Source: CAD feature listing. Evaluate the final solid. Frame: model axes, mm. A direction names the side the tool comes from. Coordinates: 2 decimals unless noted, no trailing zeros. Loops run counter-clockwise (first coordinate to the right, second up) from the corner with the lowest first, then second, coordinate; pieces in that order, holes last.
Item 1: Section query D-D, the plane z = 3. Return the cut outline in (x, y).
Item 2: Section query A-A, the plane y = -130. Return the cut outline in (x, z).
Item 3: Section query B-B, the plane x = 77. Return the cut outline in (y, z).
Item 4: Line query: probe 1 along Y at (x, z) = (110, -2.25); probe 2 along Y at (x, z) = (109.5, 4); probe 3 along X at (y, z) = (-91, 5.25). Output: solid intervals per line, ascending.
Item 5: Pin query (flat end, axial travel): pin 1 Ø2 at (y, z) = (-138, 3.5) entering from -X; pin 2 Ø3 at (x, z) = (68, -1) entering from -Y; pin 3 Ø2 at (x, z) = (124.5, -1.5) entering from +Y; pin 4 Ø0.9 at (y, z) = (-97, -1) entering from +X. Return the tip coordinate at first contact, or that it passes through.
Item 6: Reachability of faces 1 (the flat face through (2.631, -132, -1)), 2 (the flat face through (115, -136.459, 3)), 3 (the flat face through (0.631, -133, -1)), 4 (the flat face through (17, -143.959, -1)), 5 (the flat face through (128.131, -95, 3)) from +Z, -Z, +X, -X, +Y, -Y: full face, straight path, thin tool, end or side. Return the list, or none.
Item 7: Section query C-C, the plane y = -139.5. Return the cut outline in (x, z), then the cut area to 3 significant figures.
Item 8: Pull-direction query (Y, two-part tool) for faces 6 (the flat face through (13, -83.959, -1)), 7 (the flat face through (115, -116.459, 3)), 8 (the cylindrical face through (-4.307, -119.307, 3.451)); classes: +Y half, -Y half, draft (parallel to the pull), parting line (faces both ways), or undercut.
```python
from build123d import *

# Parameters (mm, degrees)
SKETCH1_W               = 29.381998836
SKETCH1_H               = 2
SKETCH1_W_2             = 22.166752634
SKETCH1_W_3             = 2
SKETCH1_H_2             = 20.351479426
SKETCH1_W_4             = 38.729480665
SKETCH1_W_5             = 32.851790847
SKETCH1_H_3             = 17.059842407
SKETCH1_H_4             = 0.5
SKETCH1_R               = 5
SKETCH1_R_2             = 1.75
BOSS_EXTRUDE1_DEPTH     = 7
BOSS_EXTRUDE3_DEPTH     = 3
CUT_EXTRUDE1_DEPTH      = 18
CUT_EXTRUDE1_DEPTH_BACK = 23
SKETCH2_R               = 8.5
SKETCH2_W               = 15
SKETCH2_H               = 20


with BuildPart() as part:
    # Sketch1 → Boss-Extrude1 (new body)
    # profile 1 of 26: a face of its own
    with BuildSketch(Plane.XY):
        Polygon((123.631337811, -141.958879214), (123.631337811, -121.052392275), (123.631337811, -103.992549868), (123.631337811, -85.958879214), (95.983128658, -85.958879214), (63.131337811, -85.958879214), (63.131337811, -141.958879214), (85.298090445, -141.958879214), align=None)
    # profile 2 of 26: a face of its own
    with BuildSketch(Plane.XY):
        Polygon((33.749338975, -141.958879214), (63.131337811, -141.958879214), (63.131337811, -85.958879214), (24.401857146, -85.958879214), (2.631337811, -85.958879214), (2.631337811, -102.239135551), (2.631337811, -122.590614977), (2.631337811, -141.958879214), align=None)
    # profile 3 of 26: a face of its own
    with BuildSketch(Plane.XY):
        with Locations((48.440338393, -142.958879214)):
            Rectangle(SKETCH1_W, SKETCH1_H)
    # profile 4 of 26: a face of its own
    with BuildSketch(Plane.XY):
        with Locations((74.214714128, -142.958879214)):
            Rectangle(SKETCH1_W_2, SKETCH1_H)
    # profile 5 of 26: a face of its own
    with BuildSketch(Plane.XY):
        Polygon((126.131337811, -144.458879214), (85.298090445, -144.458879214), (63.131337811, -144.458879214), (63.131337811, -146.458879214), (128.131337811, -146.458879214), (128.131337811, -120.364170926), (128.131337811, -113.958879254), (128.131337811, -107.553587502), (128.131337811, -81.458879214), (63.131337811, -81.458879214), (63.131337811, -83.458879214), (126.131337811, -83.458879214), align=None)
    # profile 6 of 26: a face of its own
    with BuildSketch(Plane.XY):
        Polygon((63.131337811, -146.458879214), (63.131337811, -144.458879214), (33.749338975, -144.458879214), (0.131337811, -144.458879214), (0.131337811, -102.239135551), (0.131337811, -83.458879214), (24.401857146, -83.458879214), (63.131337811, -83.458879214), (63.131337811, -81.458879214), (-1.868662189, -81.458879214), (-1.868662189, -107.553587502), (-1.868662189, -113.958879214), (-1.868662189, -120.364170926), (-1.868662189, -146.458879214), align=None)
    # profile 7 of 26: a face of its own
    with BuildSketch(Plane.XY):
        Polygon((0.631337811, -143.958879214), (33.749338975, -143.958879214), (33.749338975, -141.958879214), (2.631337811, -141.958879214), (2.631337811, -122.590614977), (0.631337811, -122.590614977), align=None)
    # profile 8 of 26: a face of its own
    with BuildSketch(Plane.XY):
        with Locations((1.631337811, -112.414875264)):
            Rectangle(SKETCH1_W_3, SKETCH1_H_2)
    # profile 9 of 26: a face of its own
    with BuildSketch(Plane.XY):
        Polygon((24.401857146, -85.958879214), (24.401857146, -83.958879214), (0.631337811, -83.958879214), (0.631337811, -102.239135551), (2.631337811, -102.239135551), (2.631337811, -85.958879214), align=None)
    # profile 10 of 26: a face of its own
    with BuildSketch(Plane.XY):
        with Locations((43.766597479, -84.958879214)):
            Rectangle(SKETCH1_W_4, SKETCH1_H)
    # profile 11 of 26: a face of its own
    with BuildSketch(Plane.XY):
        with Locations((79.557233235, -84.958879214)):
            Rectangle(SKETCH1_W_5, SKETCH1_H)
    # profile 12 of 26: a face of its own
    with BuildSketch(Plane.XY):
        Polygon((123.631337811, -103.992549868), (125.631337811, -103.992549868), (125.631337811, -83.958879214), (95.983128658, -83.958879214), (95.983128658, -85.958879214), (123.631337811, -85.958879214), align=None)
    # profile 13 of 26: a face of its own
    with BuildSketch(Plane.XY):
        with Locations((124.631337811, -112.522471072)):
            Rectangle(SKETCH1_W_3, SKETCH1_H_3)
    # profile 14 of 26: a face of its own
    with BuildSketch(Plane.XY):
        Polygon((125.631337811, -143.958879214), (125.631337811, -121.052392275), (123.631337811, -121.052392275), (123.631337811, -141.958879214), (85.298090445, -141.958879214), (85.298090445, -143.958879214), align=None)
    # profile 15 of 26: a face of its own
    with BuildSketch(Plane.XY):
        Polygon((125.631337811, -103.992549868), (125.631337811, -121.052392275), (125.631337811, -143.958879214), (85.298090445, -143.958879214), (85.298090445, -144.458879214), (126.131337811, -144.458879214), (126.131337811, -83.458879214), (63.131337811, -83.458879214), (63.131337811, -83.958879214), (95.983128658, -83.958879214), (125.631337811, -83.958879214), align=None)
    # profile 16 of 26: a face of its own
    with BuildSketch(Plane.XY):
        with Locations((74.214714128, -144.208879214)):
            Rectangle(SKETCH1_W_2, SKETCH1_H_4)
    # profile 17 of 26: a face of its own
    with BuildSketch(Plane.XY):
        with Locations((48.440338393, -144.208879214)):
            Rectangle(SKETCH1_W, SKETCH1_H_4)
    # profile 18 of 26: a face of its own
    with BuildSketch(Plane.XY):
        Polygon((33.749338975, -144.458879214), (33.749338975, -143.958879214), (0.631337811, -143.958879214), (0.631337811, -122.590614977), (0.631337811, -102.239135551), (0.131337811, -102.239135551), (0.131337811, -144.458879214), align=None)
    # profile 19 of 26: a face of its own
    with BuildSketch(Plane.XY):
        Polygon((0.631337811, -83.958879214), (24.401857146, -83.958879214), (24.401857146, -83.458879214), (0.131337811, -83.458879214), (0.131337811, -102.239135551), (0.631337811, -102.239135551), align=None)
    # profile 20 of 26: a face of its own
    with BuildSketch(Plane.XY):
        with Locations((43.766597479, -83.708879214)):
            Rectangle(SKETCH1_W_4, SKETCH1_H_4)
    # profile 21 of 26: a face of its own
    with BuildSketch(Plane.XY):
        with BuildLine():
            Line((128.131337811, -113.958879254), (128.131337811, -120.364170926))
            ThreePointArc((128.131337811, -120.364170926), (130.534472162, -119.316879015), (133.131337811, -118.958879214))
            ThreePointArc((133.131337811, -118.958879214), (129.59580392, -117.494413134), (128.131337811, -113.958879254))
        make_face()
    # profile 22 of 26: a face of its own
    with BuildSketch(Plane.XY):
        with Locations((133.131337811, -113.958879214)):
            Circle(SKETCH1_R)
        with Locations((133.131337811, -113.958879214)):
            Circle(SKETCH1_R_2, mode=Mode.SUBTRACT)
    # profile 23 of 26: a face of its own
    with BuildSketch(Plane.XY):
        with BuildLine():
            ThreePointArc((133.131337811, -108.958879214), (130.534472162, -108.600879413), (128.131337811, -107.553587502))
            Line((128.131337811, -107.553587502), (128.131337811, -113.958879254))
            ThreePointArc((128.131337811, -113.958879254), (129.595803891, -110.423345322), (133.131337811, -108.958879214))
        make_face()
    # profile 24 of 26: a face of its own
    with BuildSketch(Plane.XY):
        with Locations((-6.868662189, -113.958879214)):
            Circle(SKETCH1_R)
        with Locations((-6.868662189, -113.958879214)):
            Circle(SKETCH1_R_2, mode=Mode.SUBTRACT)
    # profile 25 of 26: a face of its own
    with BuildSketch(Plane.XY):
        with BuildLine():
            Line((-1.868662189, -113.958879214), (-1.868662189, -107.553587502))
            ThreePointArc((-1.868662189, -107.553587502), (-4.27179654, -108.600879413), (-6.868662189, -108.958879214))
            ThreePointArc((-6.868662189, -108.958879214), (-3.333128283, -110.423345308), (-1.868662189, -113.958879214))
        make_face()
    # profile 26 of 26: a face of its own
    with BuildSketch(Plane.XY):
        with BuildLine():
            ThreePointArc((-6.868662189, -118.958879214), (-4.27179654, -119.316879015), (-1.868662189, -120.364170926))
            Line((-1.868662189, -120.364170926), (-1.868662189, -113.958879214))
            ThreePointArc((-1.868662189, -113.958879214), (-3.333128283, -117.49441312), (-6.868662189, -118.958879214))
        make_face()
    extrude(amount=BOSS_EXTRUDE1_DEPTH)

    # Sketch1_4 → Boss-Extrude3 (add)
    with BuildSketch(Plane.XY):
        Polygon((123.631337811, -103.992549868), (125.631337811, -103.992549868), (125.631337811, -83.958879214), (95.983128658, -83.958879214), (95.983128658, -85.958879214), (123.631337811, -85.958879214), align=None)
        Polygon((125.631337811, -143.958879214), (125.631337811, -121.052392275), (123.631337811, -121.052392275), (123.631337811, -141.958879214), (85.298090445, -141.958879214), (85.298090445, -143.958879214), align=None)
        Polygon((0.631337811, -143.958879214), (33.749338975, -143.958879214), (33.749338975, -141.958879214), (2.631337811, -141.958879214), (2.631337811, -122.590614977), (0.631337811, -122.590614977), align=None)
        Polygon((24.401857146, -85.958879214), (24.401857146, -83.958879214), (0.631337811, -83.958879214), (0.631337811, -102.239135551), (2.631337811, -102.239135551), (2.631337811, -85.958879214), align=None)
    extrude(amount=-BOSS_EXTRUDE3_DEPTH)

    # Sketch2 → Cut-Extrude1 (cut, two sides: drawn at the far end of the back side and taken through both)
    with BuildSketch(Plane.XY.offset(7).offset(-CUT_EXTRUDE1_DEPTH_BACK)):
        with Locations((115.131337811, -96.458879214)):
            Circle(SKETCH2_R)
        with Locations((75.188241038, -96.458879214)):
            Circle(SKETCH2_R)
        with Locations((115.131337811, -126.458879214)):
            Rectangle(SKETCH2_W, SKETCH2_H)
    extrude(amount=CUT_EXTRUDE1_DEPTH + CUT_EXTRUDE1_DEPTH_BACK, mode=Mode.SUBTRACT)


solid = part.part
```
Verdict:
1. outline: (-6.87, -118.96) arc R9.6 cw to (-1.87, -120.36) - (-1.87, -146.46) - (128.13, -146.46) - (128.13, -120.36) arc R9.6 cw to (133.13, -118.96) arc R5 ccw to (133.13, -108.96) arc R9.6 cw to (128.13, -107.55) - (128.13, -81.46) - (-1.87, -81.46) - (-1.87, -107.55) arc R9.6 cw to (-6.87, -108.96) arc R5 ccw to start; hole circle Ø3.5 at (-6.87, -113.96); hole circle Ø17 at (75.19, -96.46); hole circle Ø17 at (115.13, -96.46); hole (107.63, -136.46) - (122.63, -136.46) - (122.63, -116.46) - (107.63, -116.46) - close; hole circle Ø3.5 at (133.13, -113.96)
2. outline: (-1.87, 0) - (0.63, 0) - (0.63, -3) - (2.63, -3) - (2.63, 0) - (107.63, 0) - (107.63, 7) - (-1.87, 7) - close; (122.63, 0) - (123.63, 0) - (123.63, -3) - (125.63, -3) - (125.63, 0) - (128.13, 0) - (128.13, 7) - (122.63, 7) - close
3. outline: (-146.46, 0) - (-104.76, 0) - (-104.76, 7) - (-146.46, 7) - close; (-88.15, 0) - (-81.46, 0) - (-81.46, 7) - (-88.15, 7) - close
4. probe 1: y = -143.96 to -141.96, -85.96 to -83.96
4. probe 2: y = -146.46 to -136.46, -116.46 to -102.83, -90.09 to -81.46
4. probe 3: x = -1.87 to 68.67, 81.7 to 108.62, 121.65 to 128.13
5. pin 1: stops at x = -1.87
5. pin 2: stops at y = -146.46
5. pin 3: stops at y = -83.96
5. pin 4: stops at x = 125.63
6. face 1: -Z
6. face 2: +Z, -Z
6. face 3: -Z, -X, +Y, -Y
6. face 4: -Z, +X, -X, -Y
6. face 5: +Z, -Z, +X, +Y
7. outline: (-1.87, 0) - (0.63, 0) - (0.63, -3) - (2.63, -3) - (2.63, 0) - (123.63, 0) - (123.63, -3) - (125.63, -3) - (125.63, 0) - (128.13, 0) - (128.13, 7) - (-1.87, 7) - close
7. area: 922 mm2
8. face 6: +Y half
8. face 7: undercut
8. face 8: -Y half
